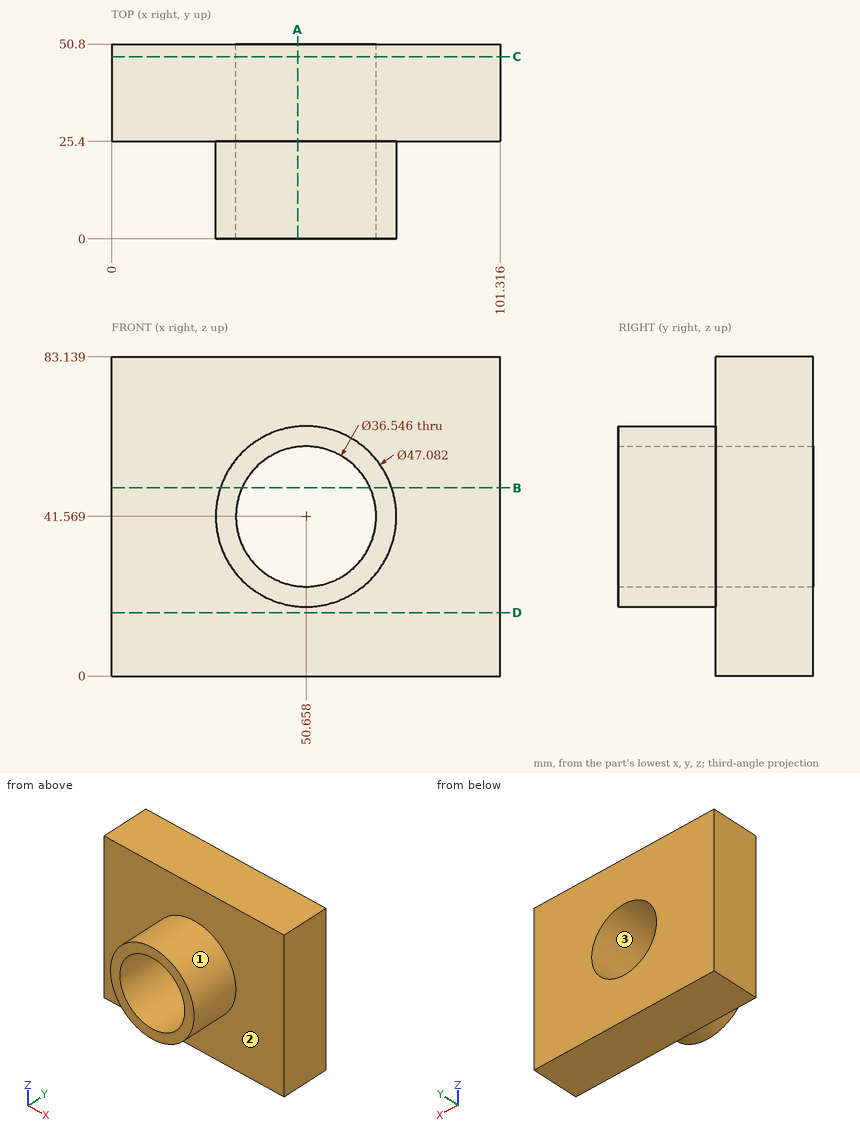
Print and shaded views of the part. All mm, measured from the part's lowest x, y and z. Give positions to 0.01 mm unless a question says otherwise; leave off trailing zeros. Loops run counter-clockwise (first coordinate to the right, second up) from the corner with the lowest first, then second, coordinate; pieces in that order, holes last. Notation, with made-up numbers: (68.5, 79.25) - (125.5, 79.25) arc R20 cw to (125.5, 118.25) - close; hole circle Ø10 at (83.25, 29.25). An arc over 180 degrees is marked (long way). One line per item, written item: value. Start each with the question number.
1. Probe L1, parallel to Z at x = 50.5, y = 38.5; L2, parallel to Z at x = 65.5, y = 35; L3, parallel to Y at x = 58.5, z = 10.5. List the from-to ranges inside material, lowest first. Write a range as from..to.
2. Pin check, flat tips, straight feed: pin 1 (12 mm diameter, centred on x = 26, y = 13, fed in from +Z) (1 decimal); pin 2 (8 mm diameter, centred on y = 29.5, z = 51, fed in from -X); pin 3 (4 mm diameter, centred on y = 22.5, z = 15, fed in from -X); pin 4 (3 mm diameter, centred on x = 57.5, z = 15.5, fed in from -Y). Stop position of each tip, or through.
3. Slice it at C-C (y = 47.5). List the corners of the cut face in (x, z) (1 decimal).
4. Slice it at A-A (x = 48.5). List the corners of the cut face in (y, z) (1 decimal), plus the area to 3 significant figures.
5. Slice it at D-D (z = 16.5). List the corners of the cut face in (x, y), plus the area to 3 significant figures.
6. Slice it at B-B (z = 49). List the corners of the cut face in (x, y) (1 decimal).
7. Pull direction Z, two halves, no side cores. Call the marked faces 1, 2 and 3: pulls with the +Z half, pulls with the -Z half, needs draft (parallel to the pull), parting line crosses it, or undercut.
Solution:
1. L1: z = 0..23.3, 59.84..83.14
1. L2: z = 0..30.91, 52.23..83.14
1. L3: y = 25.4..50.8
2. pin 1: stops at z = 55.9
2. pin 2: stops at x = 0
2. pin 3: passes through
2. pin 4: stops at y = 25.4
3. outline: (0, 0) - (101.3, 0) - (101.3, 83.1) - (0, 83.1) - close; hole circle Ø36.5 at (50.7, 41.6)
4. outline: (0, 18.1) - (25.4, 18.1) - (25.4, 0) - (50.8, 0) - (50.8, 23.4) - (0, 23.4) - close; (0, 59.7) - (50.8, 59.7) - (50.8, 83.1) - (25.4, 83.1) - (25.4, 65) - (0, 65) - close
4. area: 1,460 mm^2
5. outline: (0, 25.4) - (101.32, 25.4) - (101.32, 50.8) - (0, 50.8) - close
5. area: 2,570 mm^2
6. outline: (0, 25.4) - (28.3, 25.4) - (28.3, 0) - (34, 0) - (34, 50.8) - (0, 50.8) - close; (67.4, 0) - (73, 0) - (73, 25.4) - (101.3, 25.4) - (101.3, 50.8) - (67.4, 50.8) - close
7. face 1: parting line crosses it
7. face 2: needs draft
7. face 3: undercut
